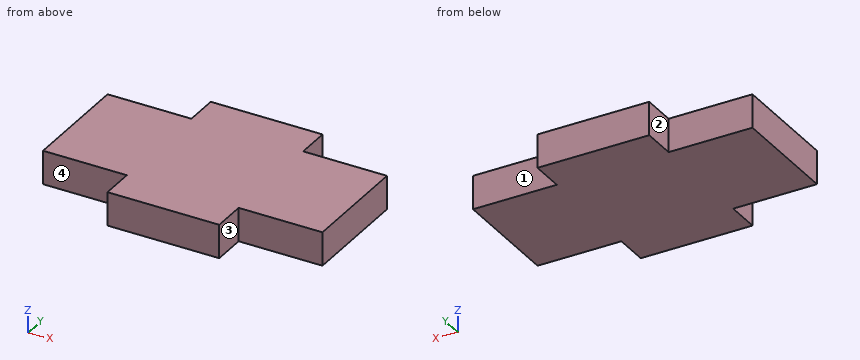
Autodesk Inventor part; units mm, degrees
ref_plane "YZ Plane" through (0, 0, 0) normal (1, 0, 0) x (0, 1, 0)
ref_plane "XZ Plane" through (0, 0, 0) normal (0, 1, 0) x (-1, 0, 0)
ref_plane "XY Plane" through (0, 0, 0) normal (0, 0, 1) x (1, 0, 0)
sketch "Boceto1" plane through (0, 0, 0) normal (0, 0, 1) x (1, 0, 0)
  line L0 (-12.5, -5) -> (-12.5, 5)
  line L1 (-5, -5) -> (-12.5, -5)
  line L2 (-5, -8) -> (-5, -5)
  line L3 (5, -8) -> (-5, -8)
  line L4 (5, -5) -> (5, -8)
  line L5 (12.5, -5) -> (5, -5)
  line L6 (12.5, 5) -> (12.5, -5)
  line L7 (5, 5) -> (12.5, 5)
  line L8 (5, 8) -> (5, 5)
  line L9 (-5, 8) -> (5, 8)
  line L10 (-5, 5) -> (-5, 8)
  line L11 (-12.5, 5) -> (-5, 5)
  point P0 (0, 0)
  point P1 (12.5, -5)
  point P2 (5, 8)
extrude "Extrusión1" add sketch "Boceto1" along normal blind 3
properties part number "Case_Support" material "MDF Tablero de fibras de densidad media"
Check sheet for the modelled part. Datum: model origin and axes. Units: mm. Face numbers are marked on the shaded views. A direction names the side the tool comes from. Coordinates: 2 decimals unless noted, no trailing zeros. Write each loop counter-clockwise with the first axis right and the second up, starting at its lowest first coordinate (ties: lowest second). Pieces come first, ordered by that corner, then holes. Notation, with made-up numbers: (21, 78) -> (78, 78) arc R18 ccw to (78, 100) -> close; hole circle Ø4 at (-23, 42). An arc over 180 degrees is marked (long way). Use a Markdown table: item, result.
1. Sectioned sample at A-A (z = 1.85). Enter the section's corners in (x, y), plus the area to 3 significant figures.
Reported:
| item | result |
|---|---|
| outline | (-12.5, -5) -> (-5, -5) -> (-5, -8) -> (5, -8) -> (5, -5) -> (12.5, -5) -> (12.5, 5) -> (5, 5) -> (5, 8) -> (-5, 8) -> (-5, 5) -> (-12.5, 5) -> close |
| area | 310 mm2 |
2. Go/stop test with flat-tipped pins: pin 1 Ø1.5 at (x, z) = (9.5, 1) entering from -Y; pin 2 Ø0.9 at (y, z) = (6, 1.5) entering from -X; pin 3 Ø1.5 at (x, z) = (7.5, 1) entering from +Y. Record where each tip stops, or that it passes through.
Reported:
| item | result |
|---|---|
| pin 1 | stops at y = -5 |
| pin 2 | stops at x = -5 |
| pin 3 | stops at y = 5 |
3. Tool access check on the marked faces 1, 2, 3 and 4. Record the directions out of +Z, -Z, +X, -X, +Y, -Y that give a thin tool (end or side, any length) a straight path to the whole face; none if there is none.
Reported:
| item | result |
|---|---|
| face 1 | +Z, -Z, +X, +Y |
| face 2 | +Z, -Z, -X, +Y |
| face 3 | +Z, -Z, +X, -Y |
| face 4 | +Z, -Z, -X, -Y |
4. Scan line: line 1 along Y through (x, z) = (-7.5, 0.65). Record every from-to range of solid material in increasing order.
Reported:
| item | result |
|---|---|
| line 1 | y = -5 to 5 |
5. Sectioned sample at B-B (y = -5.5). Enter the section's corners in (x, z), plus the area to 3 significant figures.
Reported:
| item | result |
|---|---|
| outline | (-5, 0) -> (5, 0) -> (5, 3) -> (-5, 3) -> close |
| area | 30.0 mm2 |
